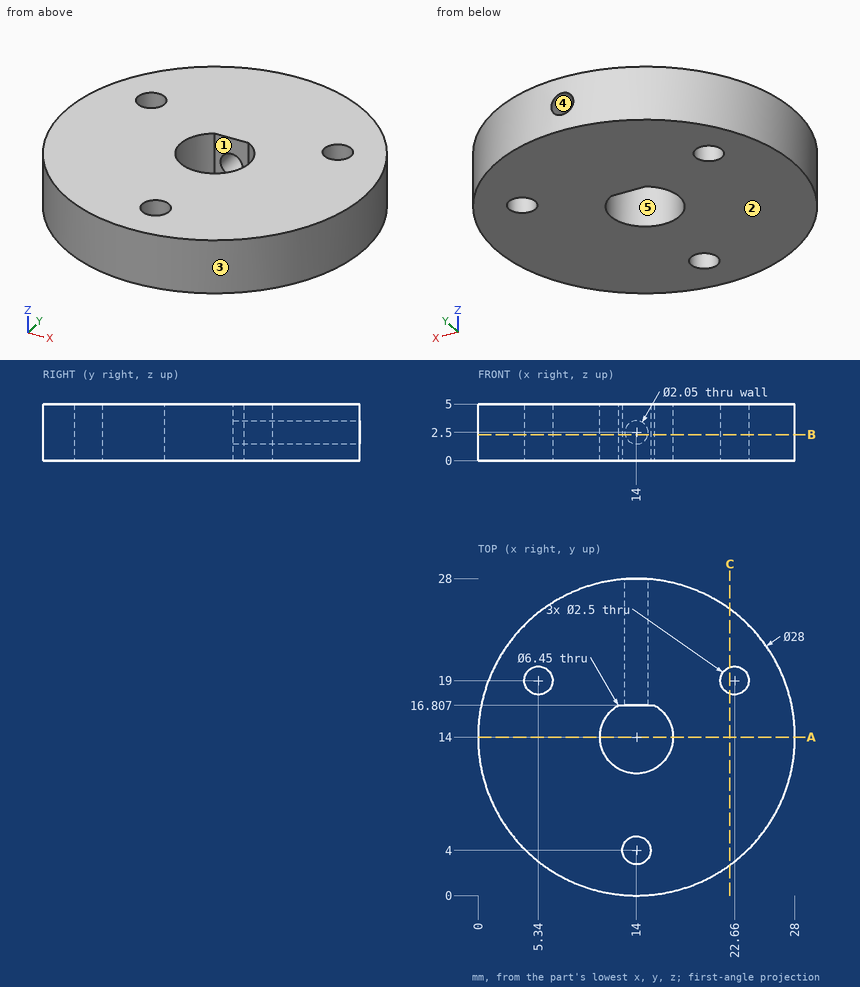
Input: dimensioned drawing with shaded views. Units: mm. Origin: part minimum x, y, z. A direction names the side the tool comes from. Give positions to 0.01 mm unless a question says otherwise; leave off trailing zeros. Write each loop counter-clockwise with the first axis right and the second up, starting at its lowest first coordinate (ties: lowest second). Pieces come first, ordered by that corner, then holes. Notation, with made-up numbers: (16, 9) - (69, 9) arc R24 ccw to (69, 34) - close; hole circle Ø5 at (12, -10.75). An arc over 180 degrees is marked (long way). One line per item, written item: value. Start each with the question number.
Q1. First-contact query: pin 1 Ø4 at (x, y) = (22.66, 19) entering from -Z; pin 2 Ø3 at (y, z) = (11.5, 4.5) entering from -X; pin 3 Ø3 at (y, z) = (7.5, 3.5) entering from +X. Flat tips, straight axial feed; report the tip coordinate or a pass-through.
Q2. Draft query along Y for the marked faces 3, 4 and 5. Return one class per face: +Y half, -Y half, draft (parallel to the pull), parting line (faces both ways), or undercut.
Q3. Material intervals for probe 1 along X at (y, z) = (3, 2); probe 2 along Y at (x, z) = (6.25, 4.05); probe 3 along Y at (x, z) = (22.25, 4.4), sorted ascending. Write a range as from..to.
Q4. Section query C-C, the plane x = 22.25. Return the cut outline in (y, z), then the cut area to 3 significant figures.
Q5. Section query B-B, the plane z = 2.3. Count the separate pieces of the cut face and the enclosed holes in it, then the cut area to 3 significant figures.
Q6. Set-up query: the marked faces 1 and 2. Return all of +Z, -Z, +X, -X, +Y, -Y with unobstructed straight access to the full face (end or side cutting, diameter ignored); none if empty.
Q7. Section query A-A, the plane y = 14. Return the cut outline in (x, z) (1 decimal), then the cut area to 3 significant figures.
Answer:
1. pin 1: stops at z = 0
1. pin 2: stops at x = 0.04
1. pin 3: stops at x = 27.08
2. face 3: parting line
2. face 4: draft
2. face 5: undercut
3. probe 1: x = 5.34..13.25, 14.75..22.66
3. probe 2: y = 2.34..18.14, 19.86..25.66
3. probe 3: y = 2.69..17.82, 20.18..25.31
4. outline: (2.69, 0) - (17.82, 0) - (17.82, 5) - (2.69, 5) - close; (20.18, 0) - (25.31, 0) - (25.31, 5) - (20.18, 5) - close
4. area: 101 mm2
5. separate pieces: 1
5. enclosed holes: 3
5. area: 547 mm2
6. face 1: +Z, -Z
6. face 2: -Z, +X, -X, +Y, -Y
7. outline: (0, 0) - (10.8, 0) - (10.8, 5) - (0, 5) - close; (17.2, 0) - (28, 0) - (28, 5) - (17.2, 5) - close
7. area: 108 mm2
